Check sheet for the modelled part. Datum: model origin and axes. Units: mm. A direction names the side the tool comes from. Give positions to 0.01 mm unless a question says otherwise; leave off trailing zeros. Loops run counter-clockwise (first coordinate to the right, second up) from the corner with the lowest first, then second, coordinate; pieces in that order, holes last. Notation, with made-up numbers: (62.25, 2.25) - (119.25, 2.25) arc R12 cw to (119.25, 6.25) - close; hole circle Ø1 at (-37, 27.5). An arc over 180 degrees is marked (long way). Answer in a Markdown table with one row per item. Add a question column.
(1) Draft check along Y on faces 1 (the face through (38.65, 9.39, -95.54)), 2 (the face through (9, 19.05, -109)), 3 (the face through (9, 0, -109)). Enter one of: released by +Y, released by -Y, zero draft, split by the parting line, or undercut.
(2) Sectioned sample at C-C on z = -125. Enter the section's corners in (x, y), then the cut area to 3 significant figures.
(3) Thickness scan on L1, parallel to X at y = 3.25, z = -9; L2, parallel to X at y = 8.25, z = -139.7; L3, parallel to Z at x = -14, y = 10.5. Record the ranges inside material, lowest first.
(4) Sectioned sample at B-B on z = -76.5. Enter the section's corners in (x, y), then the cut area to 3 significant figures.
(5) Go/stop test with flat-tipped pins: P1, Ø4, axis at x = 11.18, z = -46.58, coming from the -Y side; P2, Ø5.5, axis at x = -11, y = 13, coming from the +Z side; P3, Ø5, axis at y = 5.5, z = -159.5, coming from the +X side; P4, Ø5, axis at y = 14.5, z = -109, coming from the -X side. Record where each tip stops, or that it passes through.
(6) Sectioned sample at A-A on y = 6. State how many separate pieces and enclosed holes the cut face has, then the cut area to 3 significant figures.
(7) Set-up check for faces 4 (the face through (55.166, 9.392, -30.18)), 5 (the face through (-10, 9, -114.3)): record each of +Z, -Z, +X, -X, +Y, -Y from which the full face is reachable in a straight line by a thin tool's end or side.
from build123d import *

# Parameters (mm, degrees)
BOSS_EXTRUDE1_DEPTH              = 19.05
F_1_8_0_125_DIAMETER_HOLE1_D     = 3.175
F_1_8_0_125_DIAMETER_HOLE1_DEPTH = 11.1252
F_1_8_0_125_DIAMETER_HOLE1_TIP   = 0.953866233
F_1_8_0_125_DIAMETER_HOLE2_D     = 3.175


with BuildPart() as part:
    # Sketch1 → Boss-Extrude1 (new body)
    with BuildSketch(Plane(origin=(0, 0, 0), x_dir=(1, 0, 0), z_dir=(0, 1, 0))):
        with BuildLine():
            Line((31.75, -13.073529412), (50.765202328, 17.881902266))
            ThreePointArc((50.765202328, 17.881902266), (55.191250928, 30.365130488), (54.139291827, 43.567943639))
            Line((54.139291827, 43.567943639), (22.722603429, 148.989996692))
            ThreePointArc((22.722603429, 148.989996692), (5.710537817, 226.070917322), (0, 304.8))
            Line((0, 304.8), (-19.05, 304.8))
            Line((-19.05, 304.8), (-19.05, 114.3))
            Line((-19.05, 114.3), (0, 114.3))
            Line((0, 114.3), (0, 0))
            ThreePointArc((0, 0), (11.497376237, -17.168136702), (31.75, -13.073529412))
        make_face()
    extrude(amount=BOSS_EXTRUDE1_DEPTH)

    # 1/8 (0.125) Diameter Hole1
    with Locations(Plane(origin=(0, 0, 0), x_dir=(-1, 0, 0), z_dir=(0, -1, 0))):
        with Locations((-3.220551607, 139.7), (-18.566608997, 0), (9.525, 279.4)):
            Hole(F_1_8_0_125_DIAMETER_HOLE1_D / 2, depth=F_1_8_0_125_DIAMETER_HOLE1_DEPTH)
            with Locations((0, 0, -(F_1_8_0_125_DIAMETER_HOLE1_DEPTH + F_1_8_0_125_DIAMETER_HOLE1_TIP / 2))):  # 118° drill point
                Cone(0, F_1_8_0_125_DIAMETER_HOLE1_D / 2, F_1_8_0_125_DIAMETER_HOLE1_TIP, mode=Mode.SUBTRACT)

    # 1/8 (0.125) Diameter Hole2 (through all)
    with Locations(Plane(origin=(0, 19.05, 0), x_dir=(1, 0, 0), z_dir=(0, 1, 0))):
        with Locations((36.578180871, 46.570899758), (11.178180871, 46.576310918), (17.707917982, 9.005992113), (41.037990009, 18.900486467)):
            Hole(F_1_8_0_125_DIAMETER_HOLE2_D / 2)


solid = part.part
Reply:
| question | item | result |
|---|---|---|
| 1 | face 1 | zero draft |
| 1 | face 2 | released by +Y |
| 1 | face 3 | released by -Y |
| 2 | outline | (-19.05, 0) - (29.87, 0) - (29.87, 19.05) - (-19.05, 19.05) - close |
| 2 | area | 932 mm^2 |
| 3 | L1 | 0 to 16.12, 19.3 to 45.31 |
| 3 | L2 | -19.05 to 1.63, 4.81 to 25.49 |
| 3 | L3 | -304.8 to -114.3 |
| 4 | outline | (0, 0) - (44.33, 0) - (44.33, 19.05) - (0, 19.05) - close |
| 4 | area | 844 mm^2 |
| 5 | P1 | y = 0 |
| 5 | P2 | z = -114.3 |
| 5 | P3 | x = 20.4 |
| 5 | P4 | x = 0 |
| 6 | separate pieces | 1 |
| 6 | enclosed holes | 7 |
| 6 | area | 11,500 mm^2 |
| 7 | face 4 | +X, +Y, -Y |
| 7 | face 5 | +Z, -X, +Y, -Y |
